Geometry check sheet. Reference: the model listing, model coordinates, mm. Face numbers are marked on the shaded views. A direction names the side the tool comes from. Round coordinates to 2 decimals unless told otherwise and drop trailing zeros. Write each loop counter-clockwise with the first axis right and the second up, starting at its lowest first coordinate (ties: lowest second). Pieces come first, ordered by that corner, then holes.
Autodesk Inventor part; units mm, degrees
ref_plane "YZ Plane" through (0, 0, 0) normal (1, 0, 0) x (0, 1, 0)
ref_plane "XZ Plane" through (0, 0, 0) normal (0, 1, 0) x (-1, 0, 0)
ref_plane "XY Plane" through (0, 0, 0) normal (0, 0, 1) x (1, 0, 0)
sketch "スケッチ1" plane through (0, 0, 0) normal (1, 0, 0) x (0, 1, 0)
  line L0 (12, 0) -> (12, 5)
  line L1 (12, 5) -> (10, 5)
  line L2 (10, 5) -> (10, 10)
  line L3 (37.5, 10) -> (37.5, 0)
  line L4 (37.5, 0) -> (12, 0)
  line L5 (0, -2.4) -> (0, 14.4)
  line L6 (10, 10) -> (10, 10)
  line L7 (10, 10) -> (10, 12)
  line L8 (10, 12) -> (24, 12)
  line L9 (24, 12) -> (24, 10)
  line L10 (24, 10) -> (37.5, 10)
  point P0 (0, 0)
  dimension "d0" = 12
  dimension "d1" = 37.5
  dimension "d2" = 2
  dimension "d3" = 5
  dimension "d5" = 10
  dimension "d31" = 24
  dimension "d32" = 2
  dimension "d34" = 0
revolve "回転1" add sketch "スケッチ1" angle 360 about axis through (0, 0, -10) along (0, 0, 1)
chamfer "面取り1" distance 0.5 angle 45 1 edges at (0, -12, 0)
sketch "スケッチ2" plane through (0, 0, 10) normal (0, 0, 1) x (1, 0, 0)
  circle A0 centre (0, 0) radius 32
  point P0 (0, 32)
  point P1 (-27.7128, 16)
  point P2 (-27.7128, -16)
  point P3 (0, -32)
  point P4 (27.7128, -16)
  point P5 (27.7128, 16)
  dimension "d10" = 64
  dimension "d13" = 360
hole "穴1" at (0, 32, 10) at (-27.7128, 16, 10) at (-27.7128, -16, 10) at (0, -32, 10) at (27.7128, -16, 10) at (27.7128, 16, 10) direction (0, 0, -1) diameter 4.5 end through all
chamfer "面取り2" distance 1 angle 45 1 edges at (0, -37.5, 0)
chamfer "面取り3" distance 0.5 angle 45 1 edges at (0, -24, 12)
properties part number "unit-j2-base3" material "ABS プラスチック"
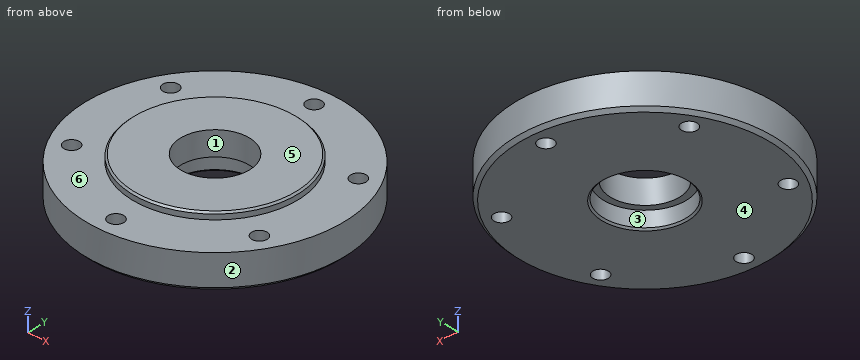
1. Section check D-D (z = 2.75). Record the cut outline in (x, y), plus the area to 3 significant figures.
2. Depth check by flat-ended pin: pin 1 Ø6 at (y, z) = (-19, 1.5) entering from +X; pin 2 Ø5 at (y, z) = (-4, 7) entering from +X; pin 3 Ø7 at (x, y) = (27.71, 16) entering from +Z. Enter the tip coordinate at first touch or a pass-through.
3. Scan lines: line 1 along Y through (x, z) = (0, 6); line 2 along Y through (x, z) = (0, 3.5); line 3 along X through (y, z) = (16.5, 1.75). Record each from-to range of solid material in increasing order.
4. Section check B-B (z = 6.75). Record the cut outline in (x, y).
5. Section check A-A (y = 0). Record the cut outline in (x, z), plus the area to 4 significant figures.
6. Access from +Z, -Z, +X, -X, +Y, -Y to the whole of each face (thin tool, end or side, straight path). Record for the marked faces 5 and 6.
7. Section check C-C (y = -16). State how many separate pieces and enclosed holes the cut face has, plus the area to 3 significant figures.
8. Release check for a two-part mould opening along X. For the marked faces 1, 2, 3 and 4 record: +X half, -X half, draft (parallel to the pull), parting line (faces both ways), or undercut.
Results below:
1. outline: circle Ø75 at (0, 0); hole circle Ø4.5 at (-27.71, -16); hole circle Ø4.5 at (-27.71, 16); hole circle Ø24 at (0, 0); hole circle Ø4.5 at (0, -32); hole circle Ø4.5 at (0, 32); hole circle Ø4.5 at (27.71, -16); hole circle Ø4.5 at (27.71, 16)
1. area: 3,870 mm2
2. pin 1: stops at x = 33.92
2. pin 2: stops at x = 37.47
2. pin 3: stops at z = 10
3. line 1: y = -37.5 to -34.25, -29.75 to -10, 10 to 29.75, 34.25 to 37.5
3. line 2: y = -37.5 to -34.25, -29.75 to -12, 12 to 29.75, 34.25 to 37.5
3. line 3: x = -33.67 to -29.91, -25.52 to 25.52, 29.91 to 33.67
4. outline: circle Ø75 at (0, 0); hole circle Ø4.5 at (-27.71, -16); hole circle Ø4.5 at (-27.71, 16); hole circle Ø20 at (0, 0); hole circle Ø4.5 at (0, -32); hole circle Ø4.5 at (0, 32); hole circle Ø4.5 at (27.71, -16); hole circle Ø4.5 at (27.71, 16)
5. outline: (-37.5, 1) - (-36.5, 0) - (-12.5, 0) - (-12, 0.5) - (-12, 5) - (-10, 5) - (-10, 12) - (-23.5, 12) - (-24, 11.5) - (-24, 10) - (-37.5, 10) - close; (10, 5) - (12, 5) - (12, 0.5) - (12.5, 0) - (36.5, 0) - (37.5, 1) - (37.5, 10) - (24, 10) - (24, 11.5) - (23.5, 12) - (10, 12) - close
5. area: 584.5 mm2
6. face 5: +Z, +X, -X, +Y, -Y
6. face 6: +Z
7. separate pieces: 3
7. enclosed holes: 0
7. area: 658 mm2
8. face 1: undercut
8. face 2: parting line
8. face 3: undercut
8. face 4: draft
